Geometry: final body of the model. Coordinates: model frame, mm. Give positions to 0.01 mm unless a question says otherwise; leave off trailing zeros. Loops run counter-clockwise (first coordinate to the right, second up) from the corner with the lowest first, then second, coordinate; pieces in that order, holes last.
from build123d import *

# Parameters (mm, degrees)
SKETCH_1_W         = 22
SKETCH_1_H         = 28
EXTRUDE_1_DEPTH    = 1.5
HOLE_WIZARD_M2_1_D = 2.4


with BuildPart() as part:
    # ｽｹｯﾁ1 → ﾎﾞｽ - 押し出し1 (new body)
    with BuildSketch(Plane.XY):
        Rectangle(SKETCH_1_W, SKETCH_1_H)
    extrude(amount=EXTRUDE_1_DEPTH)

    # M2 すきま穴1 (through all)
    with Locations(Plane.XY.offset(1.5)):
        with Locations((-9, 12), (9, 12), (-9, 1), (9, 1)):
            Hole(HOLE_WIZARD_M2_1_D / 2)


solid = part.part
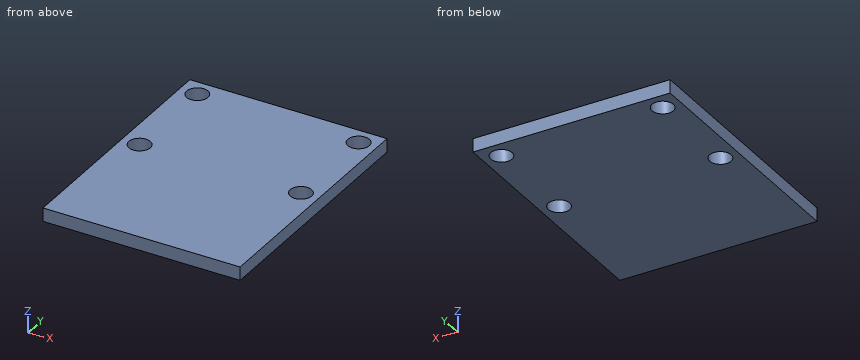
Item 1: Section query C-C on z = 1.15. Return loops of the section in (x, y), plus the area to 3 significant figures.
Values follow:
outline: (-11, -14) - (11, -14) - (11, 14) - (-11, 14) - close; hole circle Ø2.4 at (-9, 1); hole circle Ø2.4 at (-9, 12); hole circle Ø2.4 at (9, 1); hole circle Ø2.4 at (9, 12)
area: 598 mm2
Item 2: Pin query (flat end, axial travel): pin 1 (1.4 mm diameter, centred on x = 9, y = 1, fed in from +Z). Return the tip coordinate at first contact, or that it passes through.
Values follow:
pin 1: passes through
Item 3: Section query B-B on y = 1. Return loops of the section in (x, z), plus the area to 3 significant figures.
Values follow:
outline: (-11, 0) - (-10.2, 0) - (-10.2, 1.5) - (-11, 1.5) - close; (-7.8, 0) - (7.8, 0) - (7.8, 1.5) - (-7.8, 1.5) - close; (10.2, 0) - (11, 0) - (11, 1.5) - (10.2, 1.5) - close
area: 25.8 mm2
Item 4: Ray query, probe 1 along Y at (x, z) = (-9, 1.05); probe 2 along Y at (x, z) = (8.5, 1.4). Return the intervals inside material, ascending.
Values follow:
probe 1: y = -14 to -0.2, 2.2 to 10.8, 13.2 to 14
probe 2: y = -14 to -0.09, 2.09 to 10.91, 13.09 to 14
Item 5: Section query A-A on x = -9. Return loops of the section in (y, z).
Values follow:
outline: (-14, 0) - (-0.2, 0) - (-0.2, 1.5) - (-14, 1.5) - close; (2.2, 0) - (10.8, 0) - (10.8, 1.5) - (2.2, 1.5) - close; (13.2, 0) - (14, 0) - (14, 1.5) - (13.2, 1.5) - close
